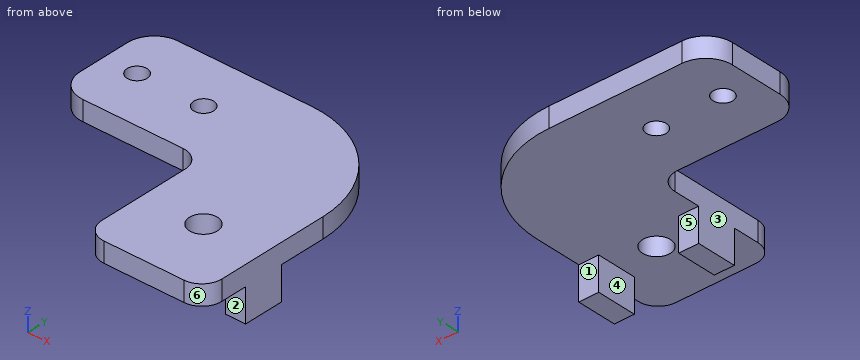
```python
from build123d import *

# Parameters (mm, degrees)
EXTRUDE_1_OUTLINE_R   = 2.1
EXTRUDE_1_OUTLINE_R_2 = 1.5
EXTRUDE_1_DEPTH       = 3
SKETCH_1_3_W          = 3
SKETCH_1_3_H          = 6
EXTRUDE_2_DEPTH       = 5


# Read off the part's stored shape, not the designer's step: the extrude step
with BuildPart() as part:
    # Extrude 1 outline → Extrude 1 (new body)
    with BuildSketch(Plane.XY):
        with BuildLine():
            ThreePointArc((41, 0), (43.121320344, 0.878679656), (44, 3))
            Line((44, 3), (44, 20))
            ThreePointArc((44, 20), (39.313708499, 31.313708499), (28, 36))
            Line((28, 36), (8, 36))
            ThreePointArc((8, 36), (5.171572875, 34.828427125), (4, 32))
            Line((4, 32), (4, 24))
            ThreePointArc((4, 24), (5.171572875, 21.171572875), (8, 20))
            Line((8, 20), (23, 20))
            ThreePointArc((23, 20), (25.121320344, 19.121320344), (26, 17))
            Line((26, 17), (26, 3))
            ThreePointArc((26, 3), (26.878679656, 0.878679656), (29, 0))
            Line((29, 0), (41, 0))
        make_face()
        with Locations((35, 10)):
            Circle(EXTRUDE_1_OUTLINE_R, mode=Mode.SUBTRACT)
        with Locations((9, 28)):
            Circle(EXTRUDE_1_OUTLINE_R_2, mode=Mode.SUBTRACT)
        with Locations((19, 28)):
            Circle(EXTRUDE_1_OUTLINE_R_2, mode=Mode.SUBTRACT)
    extrude(amount=EXTRUDE_1_DEPTH)

    # Sketch 1_3 → Extrude 2 (add)
    with BuildSketch(Plane.XY):
        with Locations((42.5, 10)):
            Rectangle(SKETCH_1_3_W, SKETCH_1_3_H)
        with Locations((27.5, 10)):
            Rectangle(SKETCH_1_3_W, SKETCH_1_3_H)
    extrude(amount=-EXTRUDE_2_DEPTH)


solid = part.part
```
CAD build for the part. Positions are in the model's coordinates, mm. Face numbers are marked on the shaded views. A direction names the side the tool comes from. Round coordinates to 2 decimals unless told otherwise and drop trailing zeros. Order: outer loops, then holes, each group sorted by start corner. A loop starts at its lowest first (then second) coordinate and runs counter-clockwise, first axis right, second up.
Q1. Two-plate mould, pull along X, no slides. Class the marked faces 4, 5 and 6: pulls with the +X half, pulls with the -X half, needs draft (parallel to the pull), parting line crosses it, or undercut.
Q2. Slice it at D-D (z = 2.25). Write the cut outline in (x, y).
Q3. Drop flat-ended pins along their axis: pin 1 (3.5 mm diameter, centred on x = 28, z = -2.5, fed in from -Y); pin 2 (2.5 mm diameter, centred on x = 18, z = 2, fed in from -Y); pin 3 (1.5 mm diameter, centred on y = 9.5, z = -2, fed in from -X); pin 4 (4 mm diameter, centred on x = 35, y = 10, fed in from +Z). Give the stop position or say it passes through.
Q4. Wall check: L1, parallel to Y at x = 19, z = 1.9; L2, parallel to Z at x = 8, y = 25; L3, parallel to Y at x = 15, z = 1. Give the ranges that are in metal, low to high.
Q5. Slice it at A-A (x = 19). Write the cut outline in (y, z).
Q6. Slice it at B-B (y = 28). Write the cut outline in (x, z).
Q7. Which spindle directions (+Z, -Z, +X, -X, +Y, -Y) get a long thin tool onto all of the face, cutting with end or side? Do the marked faces 1, 2 and 3. Say none if no direction does.
Q8. Slice it at C-C (z = -0.5). Write the cut outline in (x, y).
Results below:
1. face 4: undercut
1. face 5: needs draft
1. face 6: pulls with the +X half
2. outline: (4, 24) arc R4 ccw to (8, 20) - (23, 20) arc R3 cw to (26, 17) - (26, 3) arc R3 ccw to (29, 0) - (41, 0) arc R3 ccw to (44, 3) - (44, 20) arc R16 ccw to (28, 36) - (8, 36) arc R4 ccw to (4, 32) - close; hole circle Ø3 at (9, 28); hole circle Ø3 at (19, 28); hole circle Ø4.2 at (35, 10)
3. pin 1: stops at y = 7
3. pin 2: stops at y = 20
3. pin 3: stops at x = 26
3. pin 4: passes through
4. L1: y = 20 to 26.5, 29.5 to 36
4. L2: z = 0 to 3
4. L3: y = 20 to 36
5. outline: (20, 0) - (26.5, 0) - (26.5, 3) - (20, 3) - close; (29.5, 0) - (36, 0) - (36, 3) - (29.5, 3) - close
6. outline: (4, 0) - (7.5, 0) - (7.5, 3) - (4, 3) - close; (10.5, 0) - (17.5, 0) - (17.5, 3) - (10.5, 3) - close; (20.5, 0) - (41.86, 0) - (41.86, 3) - (20.5, 3) - close
7. face 1: -Z, +X, -X, +Y
7. face 2: -Z, +X, -X, -Y
7. face 3: +Z, -Z, -X, -Y
8. outline: (26, 7) - (29, 7) - (29, 13) - (26, 13) - close; (41, 7) - (44, 7) - (44, 13) - (41, 13) - close
